Can you work these out from the model? Positions are in its coordinate system, mm. Round coordinates to 2 decimals unless told otherwise and drop trailing zeros. Order: outer loops, then holes, each group sorted by start corner. A loop starts at its lowest first (then second) coordinate and runs counter-clockwise, first axis right, second up.
Q1. We'd pull the mould along Y, two halves only. Please class faces 1 (the face through (-161.49, -43.58, 1.52)), 2 (the face through (-140, -26.58, 1.52)): pulls with the +Y half, pulls with the -Y half, needs draft (parallel to the pull), parting line crosses it, or undercut.
Q2. If we section it at B-B (x = -171): Please give me the cut outline in (y, z).
Q3. If we section it at A-A (x = 152): Please give me the cut outline in (y, z), plus the area to 3 significant figures.
Q4. If I drill on line 1 (Y direction, x = -38, z = 2.8); line 2 (Y direction, x = 106, z = 0.8), over which ranges is the centre line in solid material (lowest first)?
Q5. If we section it at C-C (z = 1.4): Count the separate pieces of the cut face and the enclosed holes in it, plus the area to 3 significant figures.
from build123d import *

# Parameters (mm, degrees)
SKETCH_W        = 445
SKETCH_H        = 232
PAD_DEPTH       = 3
SKETCH001_R     = 9.5
POCKET_DEPTH    = 5
FILLET002_R     = 2
SKETCH015_R     = 7
POCKET009_DEPTH = 10.001


with BuildPart() as part:
    # Sketch → Pad (new body)
    with BuildSketch(Plane.XY):
        Rectangle(SKETCH_W, SKETCH_H)
    extrude(amount=PAD_DEPTH)

    # Sketch001 (on Face6 of Pad) → Pocket (cut)
    with BuildSketch(Plane.XY.offset(3)):
        with Locations((-171, 55)):
            Circle(SKETCH001_R)
        with Locations((-171, 33)):
            Circle(SKETCH001_R)
        with Locations((-171, 11)):
            Circle(SKETCH001_R)
        with Locations((-171, -11)):
            Circle(SKETCH001_R)
        with Locations((-171, -33)):
            Circle(SKETCH001_R)
        with Locations((-171, -55)):
            Circle(SKETCH001_R)
        with Locations((-152, 44)):
            Circle(SKETCH001_R)
        with Locations((-152, 22)):
            Circle(SKETCH001_R)
        with Locations((-152, 0)):
            Circle(SKETCH001_R)
        with Locations((-152, -22)):
            Circle(SKETCH001_R)
        with Locations((-152, -44)):
            Circle(SKETCH001_R)
        with Locations((-133, 55)):
            Circle(SKETCH001_R)
        with Locations((-133, 33)):
            Circle(SKETCH001_R)
        with Locations((-133, 11)):
            Circle(SKETCH001_R)
        with Locations((-133, -11)):
            Circle(SKETCH001_R)
        with Locations((-133, -33)):
            Circle(SKETCH001_R)
        with Locations((-133, -55)):
            Circle(SKETCH001_R)
        with Locations((-114, 44)):
            Circle(SKETCH001_R)
        with Locations((-114, 22)):
            Circle(SKETCH001_R)
        with Locations((-114, 0)):
            Circle(SKETCH001_R)
        with Locations((-114, -22)):
            Circle(SKETCH001_R)
        with Locations((-114, -44)):
            Circle(SKETCH001_R)
        with Locations((-95, 55)):
            Circle(SKETCH001_R)
        with Locations((-95, 33)):
            Circle(SKETCH001_R)
        with Locations((-95, 11)):
            Circle(SKETCH001_R)
        with Locations((-95, -11)):
            Circle(SKETCH001_R)
        with Locations((-95, -33)):
            Circle(SKETCH001_R)
        with Locations((-95, -55)):
            Circle(SKETCH001_R)
        with Locations((-76, -44)):
            Circle(SKETCH001_R)
        with Locations((-76, -22)):
            Circle(SKETCH001_R)
        with Locations((-76, 0)):
            Circle(SKETCH001_R)
        with Locations((-76, 22)):
            Circle(SKETCH001_R)
        with Locations((-76, 44)):
            Circle(SKETCH001_R)
        with Locations((-57, 55)):
            Circle(SKETCH001_R)
        with Locations((-57, 33)):
            Circle(SKETCH001_R)
        with Locations((-57, 11)):
            Circle(SKETCH001_R)
        with Locations((-57, -11)):
            Circle(SKETCH001_R)
        with Locations((-57, -33)):
            Circle(SKETCH001_R)
        with Locations((-38, 44)):
            Circle(SKETCH001_R)
        with Locations((-38, 22)):
            Circle(SKETCH001_R)
        with Locations((-38, 0)):
            Circle(SKETCH001_R)
        with Locations((-38, -22)):
            Circle(SKETCH001_R)
        with Locations((-38, -44)):
            Circle(SKETCH001_R)
        with Locations((-57, -55)):
            Circle(SKETCH001_R)
        with Locations((-19, 55)):
            Circle(SKETCH001_R)
        with Locations((-19, 33)):
            Circle(SKETCH001_R)
        with Locations((-19, 11)):
            Circle(SKETCH001_R)
        with Locations((-19, -11)):
            Circle(SKETCH001_R)
        with Locations((-19, -33)):
            Circle(SKETCH001_R)
        with Locations((-19, -55)):
            Circle(SKETCH001_R)
        with Locations((0, -44)):
            Circle(SKETCH001_R)
        with Locations((0, -22)):
            Circle(SKETCH001_R)
        Circle(SKETCH001_R)
        with Locations((0, 22)):
            Circle(SKETCH001_R)
        with Locations((0, 44)):
            Circle(SKETCH001_R)
        with Locations((19, 55)):
            Circle(SKETCH001_R)
        with Locations((19, 33)):
            Circle(SKETCH001_R)
        with Locations((19, 11)):
            Circle(SKETCH001_R)
        with Locations((19, -11)):
            Circle(SKETCH001_R)
        with Locations((19, -33)):
            Circle(SKETCH001_R)
        with Locations((19, -55)):
            Circle(SKETCH001_R)
        with Locations((38, -44)):
            Circle(SKETCH001_R)
        with Locations((38, -22)):
            Circle(SKETCH001_R)
        with Locations((38, 0)):
            Circle(SKETCH001_R)
        with Locations((38, 22)):
            Circle(SKETCH001_R)
        with Locations((38, 44)):
            Circle(SKETCH001_R)
        with Locations((57, 55)):
            Circle(SKETCH001_R)
        with Locations((57, 33)):
            Circle(SKETCH001_R)
        with Locations((57, 11)):
            Circle(SKETCH001_R)
        with Locations((57, -11)):
            Circle(SKETCH001_R)
        with Locations((76, 0)):
            Circle(SKETCH001_R)
        with Locations((76, 22)):
            Circle(SKETCH001_R)
        with Locations((76, 44)):
            Circle(SKETCH001_R)
        with Locations((57, -33)):
            Circle(SKETCH001_R)
        with Locations((57, -55)):
            Circle(SKETCH001_R)
        with Locations((76, -44)):
            Circle(SKETCH001_R)
        with Locations((76, -22)):
            Circle(SKETCH001_R)
        with Locations((95, 55)):
            Circle(SKETCH001_R)
        with Locations((95, 33)):
            Circle(SKETCH001_R)
        with Locations((95, 11)):
            Circle(SKETCH001_R)
        with Locations((95, -11)):
            Circle(SKETCH001_R)
        with Locations((95, -33)):
            Circle(SKETCH001_R)
        with Locations((95, -55)):
            Circle(SKETCH001_R)
        with Locations((114, 44)):
            Circle(SKETCH001_R)
        with Locations((114, 22)):
            Circle(SKETCH001_R)
        with Locations((114, 0)):
            Circle(SKETCH001_R)
        with Locations((114, -22)):
            Circle(SKETCH001_R)
        with Locations((114, -44)):
            Circle(SKETCH001_R)
        with Locations((133, 55)):
            Circle(SKETCH001_R)
        with Locations((133, 33)):
            Circle(SKETCH001_R)
        with Locations((133, 11)):
            Circle(SKETCH001_R)
        with Locations((133, -11)):
            Circle(SKETCH001_R)
        with Locations((133, -33)):
            Circle(SKETCH001_R)
        with Locations((133, -55)):
            Circle(SKETCH001_R)
        with Locations((152, 44)):
            Circle(SKETCH001_R)
        with Locations((152, 22)):
            Circle(SKETCH001_R)
        with Locations((152, 0)):
            Circle(SKETCH001_R)
        with Locations((152, -22)):
            Circle(SKETCH001_R)
        with Locations((152, -44)):
            Circle(SKETCH001_R)
        with Locations((171, 55)):
            Circle(SKETCH001_R)
        with Locations((171, 33)):
            Circle(SKETCH001_R)
        with Locations((171, 11)):
            Circle(SKETCH001_R)
        with Locations((171, -11)):
            Circle(SKETCH001_R)
        with Locations((171, -33)):
            Circle(SKETCH001_R)
        with Locations((171, -55)):
            Circle(SKETCH001_R)
    extrude(amount=-POCKET_DEPTH, mode=Mode.SUBTRACT)

    # Fillet002
    fillet002_edges = [part.edges().sort_by_distance(p)[0] for p in [
        (-222.5, -116, 1.5),
        (222.5, -116, 1.5),
        (222.5, 116, 1.5),
        (-222.5, 116, 1.5),
    ]]
    fillet(fillet002_edges, radius=FILLET002_R)

    # Sketch015 → Pocket009 (cut, through all)
    with BuildSketch(Plane.XY.offset(10)):
        with Locations((197.939534, 0)):
            Circle(SKETCH015_R)
    extrude(amount=-POCKET009_DEPTH, mode=Mode.SUBTRACT)


solid = part.part
Solution:
1. face 1: undercut
1. face 2: undercut
2. outline: (-116, 0) - (-64.5, 0) - (-64.5, 3) - (-116, 3) - close; (-45.5, 0) - (-42.5, 0) - (-42.5, 3) - (-45.5, 3) - close; (-23.5, 0) - (-20.5, 0) - (-20.5, 3) - (-23.5, 3) - close; (-1.5, 0) - (1.5, 0) - (1.5, 3) - (-1.5, 3) - close; (20.5, 0) - (23.5, 0) - (23.5, 3) - (20.5, 3) - close; (42.5, 0) - (45.5, 0) - (45.5, 3) - (42.5, 3) - close; (64.5, 0) - (116, 0) - (116, 3) - (64.5, 3) - close
3. outline: (-116, 0) - (-53.5, 0) - (-53.5, 3) - (-116, 3) - close; (-34.5, 0) - (-31.5, 0) - (-31.5, 3) - (-34.5, 3) - close; (-12.5, 0) - (-9.5, 0) - (-9.5, 3) - (-12.5, 3) - close; (9.5, 0) - (12.5, 0) - (12.5, 3) - (9.5, 3) - close; (31.5, 0) - (34.5, 0) - (34.5, 3) - (31.5, 3) - close; (53.5, 0) - (116, 0) - (116, 3) - (53.5, 3) - close
3. area: 411 mm2
4. line 1: y = -116 to -53.5, -34.5 to -31.5, -12.5 to -9.5, 9.5 to 12.5, 31.5 to 34.5, 53.5 to 116
4. line 2: y = -116 to -49.12, -38.88 to -27.12, -16.88 to -5.12, 5.12 to 16.88, 27.12 to 38.88, 49.12 to 116
5. separate pieces: 1
5. enclosed holes: 106
5. area: 73,300 mm2
